Design review of the part built by this model. Coordinates are the model's own, in mm. A direction names the side the tool comes from. Coordinates: 2 decimals unless noted, no trailing zeros. Write each loop counter-clockwise with the first axis right and the second up, starting at its lowest first coordinate (ties: lowest second). Pieces come first, ordered by that corner, then holes. Notation, with made-up numbers: (-7, 74) - (13, 74) arc R26 cw to (13, 95) - close; hole circle Ø2 at (69.25, 77.5). An arc over 180 degrees is marked (long way). Use a Markdown table: item, result.
from build123d import *

# Parameters (mm, degrees)
BOSS_EXTRUDE1_DEPTH = 562.5


with BuildPart() as part:
    # Sketch1 → Boss-Extrude1 (new, symmetric)
    with BuildSketch(Plane.XY):
        with BuildLine():
            Line((-37.5, 0), (-37.5, -50))
            ThreePointArc((-37.5, -50), (-33.838834765, -58.838834765), (-25, -62.5))
            Line((-25, -62.5), (0, -62.5))
            Line((0, -62.5), (25, -62.5))
            ThreePointArc((25, -62.5), (33.838834765, -58.838834765), (37.5, -50))
            Line((37.5, -50), (37.5, 0))
            Line((37.5, 0), (37.5, 50))
            ThreePointArc((37.5, 50), (33.838834765, 58.838834765), (25, 62.5))
            Line((25, 62.5), (-25, 62.5))
            ThreePointArc((-25, 62.5), (-33.838834765, 58.838834765), (-37.5, 50))
            Line((-37.5, 50), (-37.5, 0))
        make_face()
        with BuildLine():
            Line((-32.5, 0), (-32.5, -50))
            ThreePointArc((-32.5, -50), (-30.303300859, -55.303300859), (-25, -57.5))
            Line((-25, -57.5), (0, -57.5))
            Line((0, -57.5), (25, -57.5))
            ThreePointArc((25, -57.5), (30.303300859, -55.303300859), (32.5, -50))
            Line((32.5, -50), (32.5, 0))
            Line((32.5, 0), (32.5, 50))
            ThreePointArc((32.5, 50), (30.303300859, 55.303300859), (25, 57.5))
            Line((25, 57.5), (-25, 57.5))
            ThreePointArc((-25, 57.5), (-30.303300859, 55.303300859), (-32.5, 50))
            Line((-32.5, 50), (-32.5, 0))
        make_face(mode=Mode.SUBTRACT)
    extrude(amount=BOSS_EXTRUDE1_DEPTH, both=True)


solid = part.part
(1) For L1, parallel to Y at x = 6, z = 421; L2, parallel to X at y = -4.5, z = -414; L3, parallel to X at y = 54.5, z = -49, list the stretches that pass through material, from the lowest coordinate up. Write a range as from..to.
Determined:
| item | result |
|---|---|
| L1 | -62.5..-57.5, 57.5..62.5 |
| L2 | -37.5..-32.5, 32.5..37.5 |
| L3 | -36.66..-31, 31..36.66 |
(2) Machinability: for faces 1 (the flat face through (0, 62.5, 8)), 2 (the flat face through (0, 57.5, 8)), which of the approach directions +Z, -Z, +X, -X, +Y, -Y give a long, thin tool a straight path to every point of the face, cutting with its end or side? Answer none if there is none.
Determined:
| item | result |
|---|---|
| face 1 | +Z, -Z, +X, -X, +Y |
| face 2 | +Z, -Z |
(3) Take a section at B-B on y = -28.5. Write out the cut boundary in (x, z), and give its area (4 significant figures).
Determined:
| item | result |
|---|---|
| outline | (-37.5, -562.5) - (-32.5, -562.5) - (-32.5, 562.5) - (-37.5, 562.5) - close; (32.5, -562.5) - (37.5, -562.5) - (37.5, 562.5) - (32.5, 562.5) - close |
| area | 11,250 mm2 |
(4) Take a section at C-C on z = 229. Write out the cut boundary in (x, y).
Determined:
| item | result |
|---|---|
| outline | (-37.5, -50) arc R12.5 ccw to (-25, -62.5) - (25, -62.5) arc R12.5 ccw to (37.5, -50) - (37.5, 50) arc R12.5 ccw to (25, 62.5) - (-25, 62.5) arc R12.5 ccw to (-37.5, 50) - close; hole (-32.5, -50) arc R7.5 ccw to (-25, -57.5) - (25, -57.5) arc R7.5 ccw to (32.5, -50) - (32.5, 50) arc R7.5 ccw to (25, 57.5) - (-25, 57.5) arc R7.5 ccw to (-32.5, 50) - close |
(5) Draft analysis for pull direction Y (two halves, no side actions). For faces 3 (the flat face through (33, 0, -562.5)), 4 (the flat face through (0, -57.5, 8)), 5 (the flat face through (-32.5, 1, 8)), 6 (the flat face through (0, -62.5, 8)), state which applies: +Y half, -Y half, draft (parallel to the pull), parting line (faces both ways), or undercut.
Determined:
| item | result |
|---|---|
| face 3 | draft |
| face 4 | undercut |
| face 5 | undercut |
| face 6 | -Y half |
(6) Take a section at A-A on x = -3. Write out the cut boundary in (y, z).
Determined:
| item | result |
|---|---|
| outline | (-62.5, -562.5) - (-57.5, -562.5) - (-57.5, 562.5) - (-62.5, 562.5) - close; (57.5, -562.5) - (62.5, -562.5) - (62.5, 562.5) - (57.5, 562.5) - close |
